Design review of the part shown in the three views and the two pictorial views. Dimensions are in mm from the part's minimum x, y and z. Round coordinates to 2 decimals unless told otherwise and drop trailing zeros. Order: outer loops, then holes, each group sorted by start corner. A loop starts at its lowest first (then second) coordinate and runs counter-clockwise, first axis right, second up. Notation, with made-up numbers: M 46.5,4.5 L 93.5,4.5 A17 cw 93.5,22.5 Z; hole C 88,13.5 d11. An arc over 180 degrees is marked long. Write each question's results on one line, items separated by ' | '. Start each with the question number.
Item 1: Take a section at C-C, the plane y = 71. Write out the cut boundary in (x, z).
Item 2: Wall thickness on line 1 (X direction, y = 138.5, z = 150); line 2 (X direction, y = 272, z = 258): over which ranges is each line inside the solid? List them lowest first. Write a range as [from, to].
Item 3: Take a section at B-B, the plane x = 150. Write out the cut boundary in (y, z), plus the area to 3 significant figures.
Item 4: Take a section at A-A, the plane z = 150. Write out the cut boundary in (x, y), plus the area to 3 significant figures.
Item 5: Clearance check with flat-ended pins moving along their axes: pin 1 (1 mm diameter, centred on x = 187, y = 114, fed in from +Z); pin 2 (5 mm diameter, centred on x = 125, y = 248.5, fed in from +Z); pin 3 (7 mm diameter, centred on y = 26, z = 273.5, fed in from +X). State where each tip first meets the part, or that it passes through.
Item 6: The part is to be moulded in two halves that separate along X. For the marked faces 1 and 2, say which applies: +X half, -X half, draft (parallel to the pull), parting line (faces both ways), or undercut.
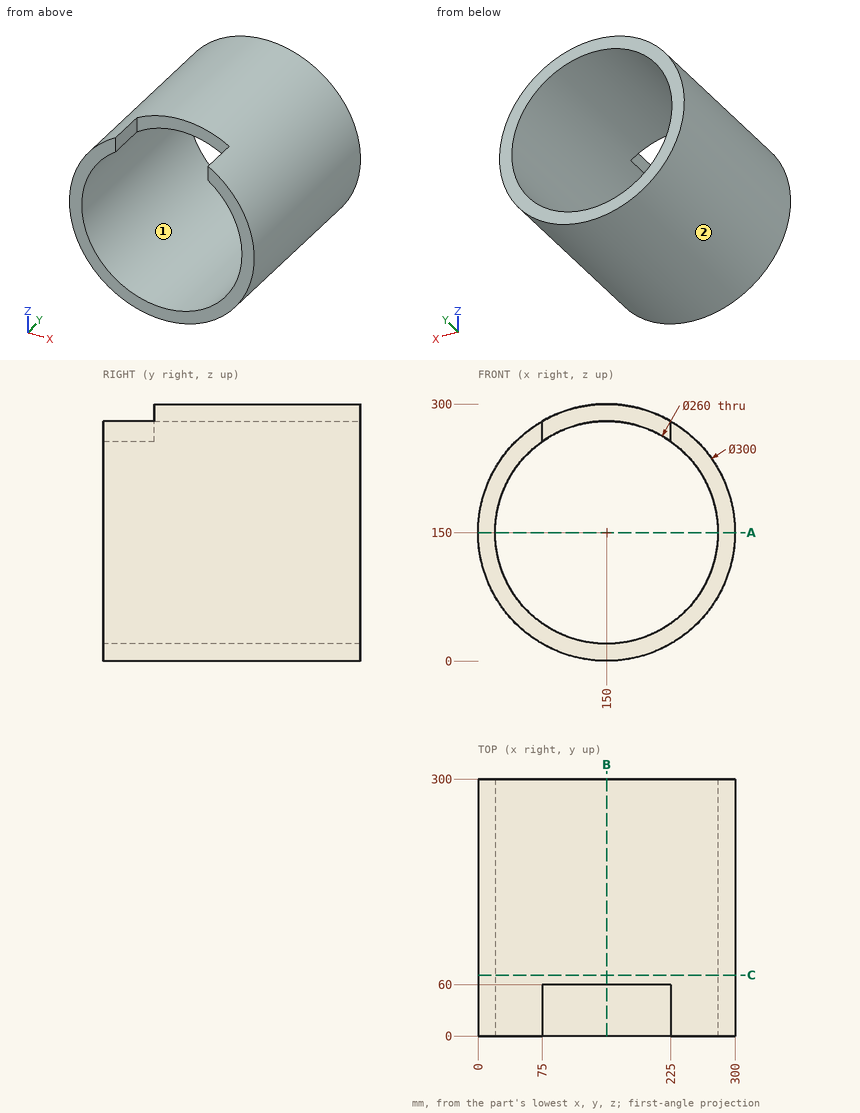
Results list:
1) outline: C 150,150 d300; hole C 150,150 d260
2) line 1: [0, 20], [280, 300] | line 2: [45.9, 77.64], [222.36, 254.1]
3) outline: M 0,0 L 300,0 L 300,20 L 0,20 Z; M 60,280 L 300,280 L 300,300 L 60,300 Z | area: 10,800 mm²
4) outline: M 0,0 L 20,0 L 20,300 L 0,300 Z; M 280,0 L 300,0 L 300,300 L 280,300 Z | area: 12,000 mm²
5) pin 1: z = 295.49 | pin 2: z = 298.3 | pin 3: x = 240
6) face 1: undercut | face 2: parting line
